Geometry: see drawing. Coordinates: mm, zero at the bounding-box minimum. A direction names the side the tool comes from. Coordinates: 2 decimals unless noted, no trailing zeros. Order: outer loops, then holes, each group sorted by start corner. A loop starts at its lowest first (then second) coordinate and runs counter-clockwise, first axis right, second up. Notation, with made-up numbers: (16, 13) -> (41, 13) arc R32 cw to (41, 40) -> close; hole circle Ø5 at (3.25, -26). An arc over 180 degrees is marked (long way). Write each question's results on one line, items separated by ' | '.
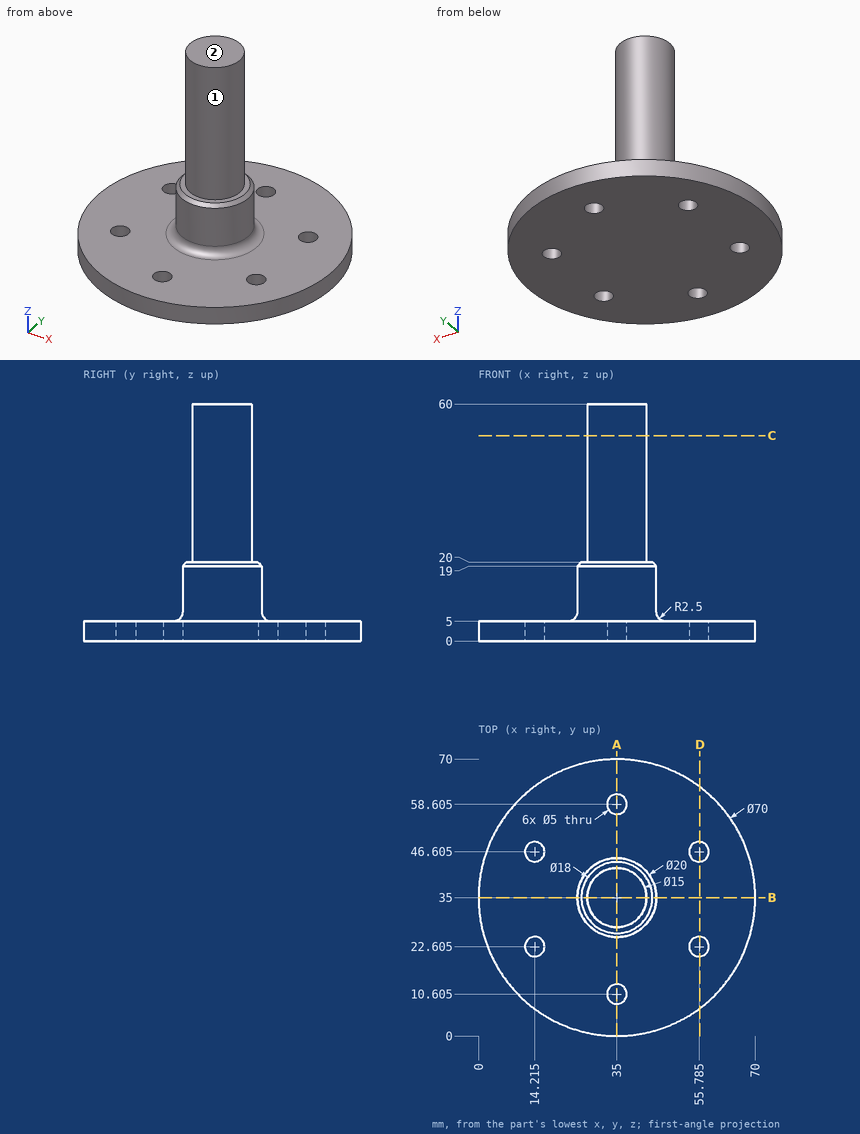
(1) Cut plane B-B, the plane y = 35. Return loops of the section in (x, z), plus the area to 3 significant figures.
Return value:
outline: (0, 0) -> (70, 0) -> (70, 5) -> (47.5, 5) arc R2.5 cw to (45, 7.5) -> (45, 19) -> (44, 20) -> (42.5, 20) -> (42.5, 60) -> (27.5, 60) -> (27.5, 20) -> (26, 20) -> (25, 19) -> (25, 7.5) arc R2.5 cw to (22.5, 5) -> (0, 5) -> close | area: 1,250 mm2
(2) Reachability of the marked faces 1 and 2 from +Z, -Z, +X, -X, +Y, -Y: full face, straight path, thin tool, end or side. Return the list, or none.
Return value:
face 1: +Z | face 2: +Z, +X, -X, +Y, -Y
(3) Line query: line 1 along Y through (x, z) = (35, 2.6) (1 decimal); line 2 along Z through (x, y) = (47, 33); line 3 along Y through (x, z) = (35.5, 22). Output: solid intervals per line, ascending. Write a range as from..to.
Return value:
line 1: 0..8.1, 13.1..56.1, 61.1..70 | line 2: 0..5.02 | line 3: 27.52..42.48
(4) Pin query (flat end, axial travel): P1, Ø6, axis at x = 35, y = 58.61, coming from the +Z side; P2, Ø8, axis at y = 41.5, z = 52, coming from the +X side; P3, Ø2, axis at y = 32, z = 53, coming from the -X side. Return the tip coordinate at first contact, or that it passes through.
Return value:
P1: z = 5 | P2: x = 42.07 | P3: x = 27.77
(5) Cut plane D-D, the plane x = 56. Return loops of the section in (y, z) (1 decimal), plus the area to 3 significant figures.
Return value:
outline: (7, 0) -> (20.1, 0) -> (20.1, 5) -> (7, 5) -> close; (25.1, 0) -> (44.1, 0) -> (44.1, 5) -> (25.1, 5) -> close; (49.1, 0) -> (63, 0) -> (63, 5) -> (49.1, 5) -> close | area: 230 mm2
(6) Cut plane A-A, the plane x = 35. Return loops of the section in (y, z) (1 decimal), plus the area to 3 significant figures.
Return value:
outline: (0, 0) -> (8.1, 0) -> (8.1, 5) -> (0, 5) -> close; (13.1, 0) -> (56.1, 0) -> (56.1, 5) -> (47.5, 5) arc R2.5 cw to (45, 7.5) -> (45, 19) -> (44, 20) -> (42.5, 20) -> (42.5, 60) -> (27.5, 60) -> (27.5, 20) -> (26, 20) -> (25, 19) -> (25, 7.5) arc R2.5 cw to (22.5, 5) -> (13.1, 5) -> close; (61.1, 0) -> (70, 0) -> (70, 5) -> (61.1, 5) -> close | area: 1,200 mm2
(7) Cut plane C-C, the plane z = 52. Return loops of the section in (x, y).
Return value:
outline: circle Ø15 at (35, 35)
